```python
from build123d import *

# Parameters (mm, degrees)
BOSS_EXTRUDE1_DEPTH = 10
SKETCH2_R           = 4
BOSS_EXTRUDE2_DEPTH = 7
BOSS_EXTRUDE3_DEPTH = 11
SKETCH5_R           = 5
BOSS_EXTRUDE4_DEPTH = 10


with BuildPart() as part:
    # Sketch1 → Boss-Extrude1 (new body)
    with BuildSketch(Plane(origin=(0, 0, 0), x_dir=(1, 0, 0), z_dir=(0, 1, 0))):
        with BuildLine():
            Line((0, -20), (95, -20))
            Line((95, -20), (95, 20))
            Line((95, 20), (0, 20))
            ThreePointArc((0, 20), (-20, 0), (0, -20))
        make_face()
        with BuildLine():
            Line((0, -5), (16.830680512, -5))
            ThreePointArc((16.830680512, -5), (21.830680512, 0), (16.830680512, 5))
            Line((16.830680512, 5), (0, 5))
            ThreePointArc((0, 5), (-5, 0), (0, -5))
        make_face(mode=Mode.SUBTRACT)
    extrude(amount=BOSS_EXTRUDE1_DEPTH)

    # Sketch2 → Boss-Extrude2 (add)
    with BuildSketch(Plane.XY.offset(20)):
        with BuildLine():
            Line((0, 10), (37, 10))
            Line((37, 10), (37, 32))
            ThreePointArc((37, 32), (29.935438849, 41.559455987), (18.723360248, 37.612239696))
            Line((18.723360248, 37.612239696), (0, 10))
        make_face()
        with Locations((27, 32)):
            Circle(SKETCH2_R, mode=Mode.SUBTRACT)
    boss_extrude2 = extrude(amount=-BOSS_EXTRUDE2_DEPTH)

    # Mirror1: Boss-Extrude2 across plane
    add(boss_extrude2.mirror(Plane.XY))

    # Sketch4 → Boss-Extrude3 (add)
    with BuildSketch(Plane(origin=(0, 10, 0), x_dir=(1, 0, 0), z_dir=(0, 1, 0))):
        Polygon((37, -20), (95, -20), (95, -10), (85, -10), (85, -15), (37, -15), align=None)
    boss_extrude3 = extrude(amount=BOSS_EXTRUDE3_DEPTH)

    # Mirror2: Boss-Extrude3 across plane
    add(boss_extrude3.mirror(Plane.XY))

    # Sketch5 → Boss-Extrude4 (add)
    with BuildSketch(Plane(origin=(95, 0, 0), x_dir=(0, 0, -1), z_dir=(1, 0, 0))):
        with BuildLine():
            Line((-10, 10), (10, 10))
            Line((10, 10), (10, 21))
            ThreePointArc((10, 21), (0, 31), (-10, 21))
            Line((-10, 21), (-10, 10))
        make_face()
        with Locations((0, 21)):
            Circle(SKETCH5_R, mode=Mode.SUBTRACT)
    extrude(amount=-BOSS_EXTRUDE4_DEPTH)


solid = part.part
```
Can you work these out from the model? Positions are in its coordinate system, mm. A direction names the side the tool comes from. Coordinates: 2 decimals unless noted, no trailing zeros. Loops run counter-clockwise (first coordinate to the right, second up) from the corner with the lowest first, then second, coordinate; pieces in that order, holes last. Notation, with made-up numbers: M 73.5,56 L 105.5,56 A5 cw 105.5,60 Z; hole C 39.5,-14.5 d10. An arc over 180 degrees is marked long. Put each result on its own line as item: value. Start each with the question number.
(1) Will these pins go through, and if not, where does the flat tip stop? pin 1 Ø6 at (y, z) = (14.5, 7) entering from -X; pin 2 Ø3 at (x, z) = (71, 15) entering from +Y; pin 3 Ø9 at (x, y) = (27, 32) entering from +Z; pin 4 Ø2 at (y, z) = (35, -13.5) entering from -X.
(2) Imagine slicing it at B-B on z = 0. List the corners of the cut face in (x, y) for me, and give its area (3 significant figures).
(3) Imagine slicing it at D-D on x = 54.5. List the corners of the cut face in (y, z) for me, and give its area (3 significant figures).
(4) I need wall thicknesses on probe 1 along Z at (x, y) = (20, 26); probe 2 along Z at (x, y) = (62, 16); probe 3 along Y at (x, z) = (91, 0). Which ranges of each line are inside material? Lowest first, please.
(5) Which directions (+Z, -Z, +X, -X, +Y, -Y) give clear straight access to the entire face, cutting with the end or side of a thin tool? Please do faces 1 (the face through (8, 5, 5)), 2 (the face through (22, 23, 13)), 3 (the face through (66, 21, 17)), 4 (the face through (37, 23, 16)), 5 (the face through (26.479, 35.966, 16.549)).
(6) Imagine slicing it at C-C on x = 27. List the corners of the cut face in (y, z) for me.
(7) We'd pull the mould along Z, two halves only. Please class faces 6 (the face through (9, 5, -5)), 7 (the face through (95, 12, 0)), 8 (the face through (-20, 5, 0)): +Z half, -Z half, draft (parallel to the pull), parting line (faces both ways), or undercut.
(8) Imagine slicing it at A-A on y = 4.5. List the corners of the cut face in (x, z) for me.
Worked answers:
1. pin 1: stops at x = 85
1. pin 2: stops at y = 21
1. pin 3: stops at z = 20
1. pin 4: stops at x = 16.27
2. outline: M -20,0 L -5,0 L -5,10 L -20,10 Z; M 21.83,0 L 95,0 L 95,16 L 85,16 L 85,10 L 21.83,10 Z; M 85,26 L 95,26 L 95,31 L 85,31 Z
2. area: 992 mm2
3. outline: M 0,-20 L 21,-20 L 21,-15 L 10,-15 L 10,15 L 21,15 L 21,20 L 0,20 Z
3. area: 510 mm2
4. probe 1: z = -20 to -13, 13 to 20
4. probe 2: z = -20 to -15, 15 to 20
4. probe 3: y = 0 to 16, 26 to 31
5. face 1: +Y, -Y
5. face 2: -X, +Y
5. face 3: +Z, +X, +Y
5. face 4: +Y
5. face 5: +Z, -Z
6. outline: M 0,-20 L 28,-20 L 28,-13 L 10,-13 L 10,13 L 28,13 L 28,20 L 0,20 Z; M 36,-20 L 42,-20 L 42,-13 L 36,-13 Z; M 36,13 L 42,13 L 42,20 L 36,20 Z
7. face 6: undercut
7. face 7: draft
7. face 8: parting line
8. outline: M 0,-20 L 95,-20 L 95,20 L 0,20 A20 ccw Z; hole M 0,-5 L 16.83,-5 A5 ccw 16.83,5 L 0,5 A5 ccw Z
